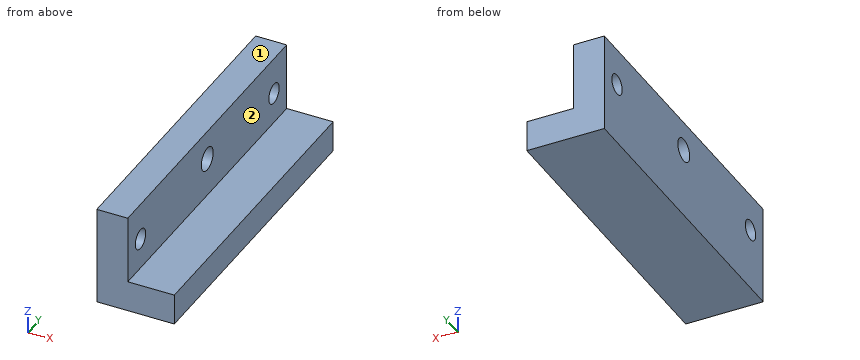
```python
from build123d import *

# Parameters (mm, degrees)
BOSS_EXTRUDE1_DEPTH        = 50
F_6_5_6_5_DIAMETER_HOLE1_D = 6.5
SKETCH4_R                  = 3.75
CUT_EXTRUDE1_DEPTH         = 65.412731661


with BuildPart() as part:
    # Sketch1 → Boss-Extrude1 (new, symmetric)
    with BuildSketch(Plane(origin=(0, 0, 0), x_dir=(1, 0, 0), z_dir=(0, 1, 0))):
        Polygon((25, 0), (0, 0), (0, -32), (10, -32), (10, -10), (25, -10), align=None)
    extrude(amount=BOSS_EXTRUDE1_DEPTH, both=True)

    # Ø6.5 (6.5) Diameter Hole1 (through all)
    with Locations(Plane.ZY):
        with Locations((20, -42), (20, 42)):
            Hole(F_6_5_6_5_DIAMETER_HOLE1_D / 2)

    # Sketch4 → Cut-Extrude1 (cut, through all)
    with BuildSketch(Plane.ZY):
        with Locations((22.5, 0)):
            Circle(SKETCH4_R)
    extrude(amount=-CUT_EXTRUDE1_DEPTH, mode=Mode.SUBTRACT)


solid = part.part
```
Here's how the part is built. I have some questions about the finished solid (model axes, mm). Face numbers are marked on the shaded views. A direction names the side the tool comes from. Give positions to 0.01 mm unless a question says otherwise; leave off trailing zeros. Order: outer loops, then holes, each group sorted by start corner. A loop starts at its lowest first (then second) coordinate and runs counter-clockwise, first axis right, second up. Notation, with made-up numbers: (77, 84.5) - (130, 84.5) arc R18 cw to (130, 111.5) - close; hole circle Ø7 at (-34.75, 2). An arc over 180 degrees is marked (long way). Answer as a JSON object with one key per item and string values. Group by question number.
Item 1: If we section it at D-D on z = 20: Please give me the cut outline in (x, y).
Item 2: If we section it at A-A on y = 0: Please give me the cut outline in (x, z).
Item 3: If we section it at B-B on x = 5: Please give me the cut outline in (y, z), and give its area (3 significant figures).
Item 4: For P1, Ø3, axis at y = -2.5, z = 23.5, coming from the +X side; P2, Ø4.5, axis at x = 18.5, y = 10, coming from the +Z side, each with a flat end and sliding along its axis, tell me the tip position at first contact or that it passes through.
Item 5: Please list where these lines run through material, in increasing order: probe 1 along Y at (x, z) = (4.5, 22.5); probe 2 along Y at (x, z) = (4.25, 20); probe 3 along Z at (x, y) = (18.25, -19.5).
Item 6: If we section it at C-C on y = 42: Please give me the cut outline in (x, z), and give its area (3 significant figures).
Item 7: Which directions (+Z, -Z, +X, -X, +Y, -Y) give clear straight access to the entire face, cutting with the end or side of a thin tool? Please do the marked faces 1 and 2.
Result set:
{
 "1": {"outline": "(0, -50) - (10, -50) - (10, -45.25) - (0, -45.25) - close; (0, -38.75) - (10, -38.75) - (10, -2.8) - (0, -2.8) - close; (0, 2.8) - (10, 2.8) - (10, 38.75) - (0, 38.75) - close; (0, 45.25) - (10, 45.25) - (10, 50) - (0, 50) - close"},
 "2": {"outline": "(0, 0) - (25, 0) - (25, 10) - (10, 10) - (10, 18.75) - (0, 18.75) - close; (0, 26.25) - (10, 26.25) - (10, 32) - (0, 32) - close"},
 "3": {"outline": "(-50, 0) - (50, 0) - (50, 32) - (-50, 32) - close; hole circle Ø6.5 at (-42, 20); hole circle Ø7.5 at (0, 22.5); hole circle Ø6.5 at (42, 20)", "area": "3,090 mm²"},
 "4": {"P1": "x = 10", "P2": "z = 10"},
 "5": {"probe 1": "-50 to -44.08, -39.92 to -3.75, 3.75 to 39.92, 44.08 to 50", "probe 2": "-50 to -45.25, -38.75 to -2.8, 2.8 to 38.75, 45.25 to 50", "probe 3": "0 to 10"},
 "6": {"outline": "(0, 0) - (25, 0) - (25, 10) - (10, 10) - (10, 16.75) - (0, 16.75) - close; (0, 23.25) - (10, 23.25) - (10, 32) - (0, 32) - close", "area": "405 mm²"},
 "7": {"face 1": "+Z, +X, -X, +Y, -Y", "face 2": "+Z, +X, +Y, -Y"}
}
